```python
from build123d import *

# Parameters (mm, degrees)
BOSS_EXTRUDE1_DEPTH = 15
CUT_EXTRUDE1_DEPTH  = 17.439282223
CUT_EXTRUDE2_START  = -4.5
SKETCH3_W           = 10
SKETCH3_H           = 5.3
CUT_EXTRUDE2_DEPTH  = 2
SKETCH4_W           = 3
SKETCH4_H           = 0.815561475
CUT_EXTRUDE3_DEPTH  = 2
CHAMFER1_SIZE       = 1.5


with BuildPart() as part:
    # Sketch1 → Boss-Extrude1 (new body)
    with BuildSketch(Plane.XY):
        with BuildLine():
            Line((0, 0), (-4, 0))
            ThreePointArc((-4, 0), (-4.707106781, 0.292893219), (-5, 1))
            Line((-5, 1), (-5, 2.5))
            ThreePointArc((-5, 2.5), (-3, 4.5), (-1, 2.5))
            Line((-1, 2.5), (-1, 1.3))
            Line((-1, 1.3), (-1.5, 1.3))
            Line((-1.5, 1.3), (-1.5, 2.5))
            ThreePointArc((-1.5, 2.5), (-3, 4), (-4.5, 2.5))
            Line((-4.5, 2.5), (-4.5, 1))
            ThreePointArc((-4.5, 1), (-4.353553391, 0.646446609), (-4, 0.5))
            Line((-4, 0.5), (0, 0.5))
            Line((0, 0.5), (4, 0.5))
            ThreePointArc((4, 0.5), (4.353553391, 0.646446609), (4.5, 1))
            Line((4.5, 1), (4.5, 2.5))
            ThreePointArc((4.5, 2.5), (3, 4), (1.5, 2.5))
            Line((1.5, 2.5), (1.5, 1.3))
            Line((1.5, 1.3), (1, 1.3))
            Line((1, 1.3), (1, 2.5))
            ThreePointArc((1, 2.5), (3, 4.5), (5, 2.5))
            Line((5, 2.5), (5, 1))
            ThreePointArc((5, 1), (4.707106781, 0.292893219), (4, 0))
            Line((4, 0), (0, 0))
        make_face()
    extrude(amount=-BOSS_EXTRUDE1_DEPTH)

    # Sketch2 → Cut-Extrude1 (cut, through all)
    with BuildSketch(Plane.XZ):
        with BuildLine():
            Line((-4, 0), (-2.4, -1.6))
            Line((-2.4, -1.6), (-2.4, -4))
            ThreePointArc((-2.4, -4), (-1.5, -4.9), (-0.6, -4))
            Line((-0.6, -4), (0.6, -4))
            ThreePointArc((0.6, -4), (1.5, -4.9), (2.4, -4))
            Line((2.4, -4), (2.4, -1.6))
            Line((2.4, -1.6), (4, 0))
            Line((4, 0), (4, 0.537500588))
            Line((4, 0.537500588), (-4, 0.537500588))
            Line((-4, 0.537500588), (-4, 0))
        make_face()
    extrude(amount=-CUT_EXTRUDE1_DEPTH, mode=Mode.SUBTRACT)

    # Sketch3 → Cut-Extrude2 (cut)
    with BuildSketch(Plane.XZ.offset(CUT_EXTRUDE2_START)):
        with Locations((0, -2.65)):
            Rectangle(SKETCH3_W, SKETCH3_H)
    extrude(amount=CUT_EXTRUDE2_DEPTH, mode=Mode.SUBTRACT)

    # Sketch4 → Cut-Extrude3 (cut)
    with BuildSketch(Plane(origin=(0, 2.5, 0), x_dir=(1, 0, 0), z_dir=(0, 1, 0))):
        with Locations((0, 4.892219263)):
            Rectangle(SKETCH4_W, SKETCH4_H)
    extrude(amount=-CUT_EXTRUDE3_DEPTH, mode=Mode.SUBTRACT)

    # Chamfer1
    chamfer1_edges = [part.edges().sort_by_distance(p)[0] for p in [
        (4.75, 2.5, 0),
        (-4.75, 2.5, 0),
        (1.25, 1.3, -15),
        (-1.25, 1.3, -15),
    ]]
    chamfer(chamfer1_edges, length=CHAMFER1_SIZE)


solid = part.part
```
Model file for the job. Use its own axes, mm. A direction names the side the tool comes from. Coordinates: 2 decimals unless noted, no trailing zeros. Write each loop counter-clockwise with the first axis right and the second up, starting at its lowest first coordinate (ties: lowest second). Pieces come first, ordered by that corner, then holes. Notation, with made-up numbers: (33, 89) - (63, 89) arc R13 cw to (63, 104) - close; hole circle Ø2 at (54, 27). An arc over 180 degrees is marked (long way). Use a Markdown table: item, result. Add a question column.
Item 1: 3-axis set-ups, long thin cutter, end or side, ignore diameter. For faces 5 (the face through (-1.5, 2, -10)), 6 (the face through (-3.2, 0.2, -0.8)), 7 (the face through (-1, 2, -10)), 8 (the face through (-4.699, 0.285, -7.395)), 9 (the face through (-1.458, 3.094, -15)): which of +Z, -Z, +X, -X, +Y, -Y reach the whole face in a straight line?
Item 2: Drop flat-ended pins along their axis: pin 1 (0.6 mm diameter, centred on x = 4.5, z = -3, fed in from +Y); pin 2 (2.5 mm diameter, centred on x = -0.5, z = -9, fed in from +Y); pin 3 (1 mm diameter, centred on y = 4, z = -5.5, fed in from -X). Give the stop position or say it passes through.
Item 3: Drill centre lines: line 1 along X through (y, z) = (1.6, -8); line 2 along X through (y, z) = (3.1, -13); line 3 along Z through (x, y) = (-4, 3.9). Where is each one in solid material? Low to high.
Item 4: Band-saw the part on C-C, the plane z = -11. Write the cut outline in (x, y), and give its area (3 significant figures).
Item 5: Band-saw the part on A-A, the plane x = -3. Write the cut outline in (y, z), and give its area (4 significant figures).
Item 6: Band-saw the part on D-D, the plane y = 0.8. Write the cut outline in (x, z).
Item 7: Band-saw the part on B-B, the plane y = 3.7. Write the cut outline in (x, z), and give its area (3 significant figures).
Item 8: Two-plate mould, pull along Y, no slides. Class faces 1 (the face through (3.2, 0.2, -0.8)), 2 (the face through (-1.3, 2, -14.2)), 3 (the face through (4.715, 0.301, -7.395)), 4 (the face through (4.7, 1.8, -0.8)): pulls with the +Y half, pulls with the -Y half, needs draft (parallel to the pull), parting line crosses it, or undercut.
A:
| question | item | result |
|---|---|---|
| 1 | face 5 | +Z, -Z |
| 1 | face 6 | +Z, +Y, -Y |
| 1 | face 7 | +Z, -Z, +Y |
| 1 | face 8 | +Z, -Z, -X, -Y |
| 1 | face 9 | -Z, +X, -X, +Y, -Y |
| 2 | pin 1 | stops at y = 2.5 |
| 2 | pin 2 | stops at y = 4.06 |
| 2 | pin 3 | stops at x = -4.73 |
| 3 | line 1 | x = -5 to -4.5, -1.5 to -1, 1 to 1.5, 4.5 to 5 |
| 3 | line 2 | x = -4.91 to -4.37, -1.63 to -1.09, 1.09 to 1.63, 4.37 to 4.91 |
| 3 | line 3 | z = -15 to -5.3 |
| 4 | outline | (-5, 1) arc R1 ccw to (-4, 0) - (4, 0) arc R1 ccw to (5, 1) - (5, 2.5) arc R2 ccw to (1, 2.5) - (1, 1.3) - (1.5, 1.3) - (1.5, 2.5) arc R1.5 cw to (4.5, 2.5) - (4.5, 1) arc R0.5 cw to (4, 0.5) - (-4, 0.5) arc R0.5 cw to (-4.5, 1) - (-4.5, 2.5) arc R1.5 cw to (-1.5, 2.5) - (-1.5, 1.3) - (-1, 1.3) - (-1, 2.5) arc R2 ccw to (-5, 2.5) - close |
| 4 | area | 13.4 mm² |
| 5 | outline | (0, -15) - (0.5, -15) - (0.5, -1) - (0, -1) - close; (4, -15) - (4.5, -15) - (4.5, -5.3) - (4, -5.3) - close |
| 5 | area | 11.85 mm² |
| 6 | outline | (-4.98, -15) - (-4.46, -15) - (-4.46, 0) - (-4.98, 0) - close; (4.46, -15) - (4.98, -15) - (4.98, 0) - (4.46, 0) - close |
| 7 | outline | (-4.6, -15) - (-3.9, -15) - (-3.9, -5.3) - (-4.6, -5.3) - close; (-2.1, -15) - (-1.4, -15) - (-1.4, -5.3) - (-2.1, -5.3) - close; (1.4, -15) - (2.1, -15) - (2.1, -5.3) - (1.4, -5.3) - close; (3.9, -15) - (4.6, -15) - (4.6, -5.3) - (3.9, -5.3) - close |
| 7 | area | 27.2 mm² |
| 8 | face 1 | needs draft |
| 8 | face 2 | undercut |
| 8 | face 3 | pulls with the -Y half |
| 8 | face 4 | pulls with the +Y half |
